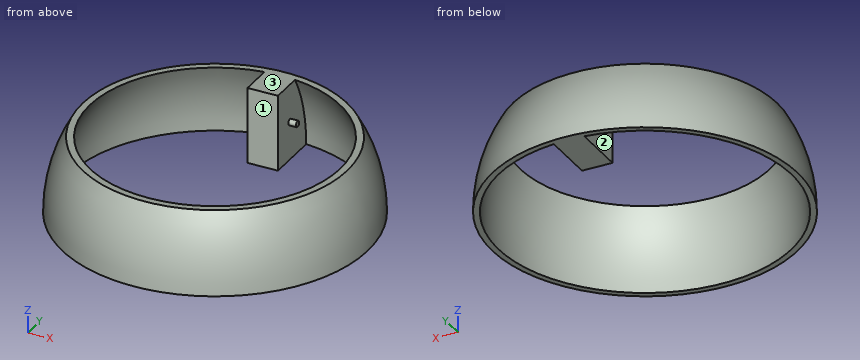
```python
from build123d import *

# Parameters (mm, degrees)
F2_T     = -4
F4_W     = 20
F4_H     = 50
F5_REACH = 93.8526480713
F6_R     = 2
F7_DEPTH = 5


with BuildPart() as f1:
    # F0 (on Front) → F1 (revolve)
    with BuildSketch(Plane.XZ):
        with BuildLine():
            Line((0, 0), (100, 0))
            ThreePointArc((100, 0), (96.5925826289, 25.8819045103), (86.6025403784, 50))
            Line((86.6025403784, 50), (0, 50))
            Line((0, 50), (0, 0))
        make_face()
    revolve(axis=Axis((0, 0, 53.0949570239), (0, 0, 1)))

    # F2
    f2_openings = [f1.faces().sort_by_distance(p)[0] for p in [
        (0, 0, 0),
        (0, 0, 50),
    ]]
    offset(amount=F2_T, openings=f2_openings)

    f5_end = f1.faces().sort_by_distance((-96.5925826289, 0, 25.8819045103))[0]
    # F4 (on offset) → F5 (join, up to a face of the model that its end follows)
    with BuildSketch(Plane.XZ.offset(-60)):
        with Locations((0, 25)):
            Rectangle(F4_W, F4_H)
    f5_long = extrude(amount=-F5_REACH, mode=Mode.PRIVATE)
    add(split(f5_long, bisect_by=f5_end, keep=Keep.BOTTOM, mode=Mode.PRIVATE))

    # F6 (on face) → F7 (join)
    with BuildSketch(Plane.YZ.offset(10)):
        with Locations((75, 25)):
            Circle(F6_R)
    extrude(amount=F7_DEPTH)


solid = f1.part
```
Design review of the part built by this model. Coordinates are the model's own, in mm. Face numbers are marked on the shaded views. A direction names the side the tool comes from. Give positions to 0.01 mm unless a question says otherwise; leave off trailing zeros. Write each loop counter-clockwise with the first axis right and the second up, starting at its lowest first coordinate (ties: lowest second). Pieces come first, ordered by that corner, then holes. Notation, with made-up numbers: (83, -31) - (95, -31) arc R21 cw to (95, -22) - close; hole circle Ø11 at (-4, 65.5). An arc over 180 degrees is marked (long way). Return JSON: item names as keys, results as strings. Group by question number.
(1) We need section B-B, the plane y = 22.5. Give the boundary of the cut face in (x, z).
(2) Insertion check: pin 1 (8 mm diameter, centred on x = -8, z = 40.5, fed in from +Y); pin 2 (10 mm diameter, centred on x = 71, z = 21, fed in from -Y); pin 3 (6 mm diameter, centred on x = -33.5, z = 21.5, fed in from -Y); pin 4 (8 mm diameter, centred on x = -75, y = -17.5, fed in from +Z). Each pin has a flat end and moves straight along its axis. Give the tip position at first contact, or say it passes through.
(3) We need section A-A, the plane x = 41.5. Give the boundary of the cut face in (y, z).
(4) To check wall thickness, follow probe 1 along X at (y, z) = (70, 12); probe 2 along X at (y, z) = (75, 45.5); probe 3 along Y at (x, z) = (79, 9). State the ranges of each line that lie inside material, in increasing order.
(5) Machinability: for the marked faces 1, 2 and 3, which of the approach directions +Z, -Z, +X, -X, +Y, -Y give a long, thin tool a straight path to every point of the face, cutting with its end or side? Answer none if there is none.
Reported:
{
 "1": {"outline": "(-97.44, 0) - (-93.33, 0) arc R93.33 cw to (-78.8, 50) - (-83.63, 50) arc R97.44 ccw to start; (78.8, 50) arc R93.33 cw to (93.33, 0) - (97.44, 0) arc R97.44 ccw to (83.63, 50) - close"},
 "2": {"pin 1": "stops at y = 92.79", "pin 2": "stops at y = -72.34", "pin 3": "stops at y = -92.98", "pin 4": "passes through"},
 "3": {"outline": "(-90.98, 0) - (-86.57, 0) arc R86.57 cw to (-70.67, 50) - (-76.01, 50) arc R90.98 ccw to start; (70.67, 50) arc R86.57 cw to (86.57, 0) - (90.98, 0) arc R90.98 ccw to (76.01, 50) - close"},
 "4": {"probe 1": "x = -70.4 to -64.59, -10 to 10, 64.59 to 70.4", "probe 2": "x = -48.01 to -39, -10 to 10, 39 to 48.01", "probe 3": "y = -60.65 to -53.8, 53.8 to 60.65"},
 "5": {"face 1": "+Z, -Z", "face 2": "-Z", "face 3": "+Z, +X, -X, +Y, -Y"}
}
